Can you work these out from the model? Positions are in its coordinate system, mm. Face numbers are marked on the shaded views. A direction names the side the tool comes from. Give positions to 0.01 mm unless a question says otherwise; leave off trailing zeros. Loops run counter-clockwise (first coordinate to the right, second up) from the corner with the lowest first, then second, coordinate; pieces in that order, holes last. Notation, with made-up numbers: M -8.75,-20.5 L 49.25,-20.5 A8 cw 49.25,-9.5 Z; hole C -16.75,-0.75 d3. An arc over 180 degrees is marked long. Put each result on its own line as item: value. Start each with the question number.
1) For P1, Ø10, axis at x = 33.5, y = -88, coming from the -Z side; P2, Ø2, axis at y = -81, z = -4, coming from the +X side; P3, Ø12, axis at x = 117.5, z = 5, coming from the +Y side, each with a flat end and sliding along its axis, tell me the tip position at first contact or that it passes through.
2) Please list where these lines run through material, in increasing order: line 1 along X through (y, z) = (-70.25, 12.5); line 2 along X through (y, z) = (-75, 9); line 3 along Y through (x, z) = (90.5, 1). Write a range as from..to.
3) For the marked faces 5, 6 and 7, which set-ups out of +Z, -Z, +X, -X, +Y, -Y let a thin tool reach every point of the face, with its end or its side?
4) Imagine slicing it at C-C (x = 95). Write out the boundary of the cut face in (y, z), then the cut area to 3 significant figures.
5) Imagine slicing it at A-A (z = 12.5). Write out the boundary of the cut face in (x, y).
6) Imagine slicing it at B-B (z = -7). Write out the boundary of the cut face in (x, y).
7) If we mould it in two halves opening along Y, with no side actions, what happens to the marked faces 1, 2, 3 and 4? For each: +Y half, -Y half, draft (parallel to the pull), parting line (faces both ways), or undercut.
from build123d import *

# Parameters (mm, degrees)
SKETCH_1_W          = 170
SKETCH_1_H          = 150
EXTRUDE_1_DEPTH     = 25
CUT_EXTRUDE_1_DEPTH = 50
CHAMFER_2_SIZE      = 5
SKETCH_7_R          = 6
EXTRUDE_4_DEPTH     = 10
CHAMFER_4_SIZE      = 5
SKETCH_8_R          = 5
CUT_EXTRUDE_2_DEPTH = 229.089894559


with BuildPart() as part:
    # 草图1 → 凸台-拉伸1 (new body)
    with BuildSketch(Plane.XY):
        with Locations((85, -75)):
            Rectangle(SKETCH_1_W, SKETCH_1_H)
    extrude(amount=EXTRUDE_1_DEPTH)

    # 草图3 → 切除-拉伸1 (cut)
    with BuildSketch(Plane(origin=(0, 0, 0), x_dir=(-1, 0, 0), z_dir=(0, 0, -1))):
        with BuildLine():
            Line((-170, 0), (-105, 0))
            ThreePointArc((-105, 0), (-215.961940777, 45.961940777), (-170, -65))
            Line((-170, -65), (-170, 0))
        make_face()
        with BuildLine():
            ThreePointArc((-170, -65), (-124.038059223, -45.961940777), (-105, 0))
            Line((-105, 0), (-170, 0))
            Line((-170, 0), (-170, -65))
        make_face()
        with BuildLine():
            ThreePointArc((0, -61.846584384), (18.242646352, 52.559490104), (-85, 0))
            Line((-85, 0), (-20, 0))
            Line((-20, 0), (0, 0))
            Line((0, 0), (0, -61.846584384))
        make_face()
        with BuildLine():
            Line((-20, 0), (-85, 0))
            ThreePointArc((-85, 0), (-65.961940777, -45.961940777), (-20, -65))
            Line((-20, -65), (0, -65))
            Line((0, -65), (0, -61.846584384))
            Line((0, -61.846584384), (0, 0))
            Line((0, 0), (-20, 0))
        make_face()
        with BuildLine():
            Line((0, -150), (-85, -150))
            ThreePointArc((-85, -150), (18.242646352, -202.559490104), (0, -88.153415616))
            Line((0, -88.153415616), (0, -150))
        make_face()
        with BuildLine():
            Line((0, -88.153415616), (0, -85))
            Line((0, -85), (-20, -85))
            ThreePointArc((-20, -85), (-65.961940777, -104.038059223), (-85, -150))
            Line((-85, -150), (0, -150))
            Line((0, -150), (0, -88.153415616))
        make_face()
        with BuildLine():
            Line((-170, -150), (-170, -85))
            ThreePointArc((-170, -85), (-215.961940777, -195.961940777), (-105, -150))
            Line((-105, -150), (-170, -150))
        make_face()
        with BuildLine():
            ThreePointArc((-105, -150), (-124.038059223, -104.038059223), (-170, -85))
            Line((-170, -85), (-170, -150))
            Line((-170, -150), (-105, -150))
        make_face()
    extrude(amount=-CUT_EXTRUDE_1_DEPTH, mode=Mode.SUBTRACT)

    # 倒角2
    chamfer_2_edges = [part.edges().sort_by_distance(p)[0] for p in [
        (0, -75, 0),
        (95, 0, 0),
        (170, -75, 0),
        (95, -150, 0),
        (124.038059223, -45.961940777, 0),
        (65.961940777, -45.961940777, 0),
        (124.038059223, -104.038059223, 0),
        (65.961940777, -104.038059223, 0),
        (10, -85, 0),
        (10, -65, 0),
    ]]
    chamfer(chamfer_2_edges, length=CHAMFER_2_SIZE)

    # 草图7 → 凸台-拉伸4 (add)
    with BuildSketch(Plane(origin=(0, 0, 0), x_dir=(-1, 0, 0), z_dir=(0, 0, -1))):
        with Locations(Location((-107.5, -62.5, 0), (0, 0, 180))):
            Circle(SKETCH_7_R)
        with Locations(Location((-82.5, -62.5, 0), (0, 0, 180))):
            Circle(SKETCH_7_R)
        with Locations(Location((-82.5, -87.5, 0), (0, 0, 180))):
            Circle(SKETCH_7_R)
        with Locations(Location((-107.5, -87.5, 0), (0, 0, 180))):
            Circle(SKETCH_7_R)
    extrude(amount=EXTRUDE_4_DEPTH)

    # 倒角4
    chamfer_4_edges = [part.edges().sort_by_distance(p)[0] for p in [
        (0, -75, 25),
        (95, -150, 25),
        (170, -75, 25),
        (95, 0, 25),
        (124.038059223, -104.038059223, 25),
        (10, -85, 25),
        (65.961940777, -104.038059223, 25),
        (10, -65, 25),
        (65.961940777, -45.961940777, 25),
        (124.038059223, -45.961940777, 25),
    ]]
    chamfer(chamfer_4_edges, length=CHAMFER_4_SIZE)

    # 草图8 → 切除-拉伸2 (cut, through all)
    with BuildSketch(Plane(origin=(0, 0, 0), x_dir=(1, 0, 0), z_dir=(0, 1, 0))):
        with Locations(Location((20, -12.5, 0), (0, 0, 270))):
            Circle(SKETCH_8_R)
    extrude(amount=-CUT_EXTRUDE_2_DEPTH, mode=Mode.SUBTRACT)


solid = part.part
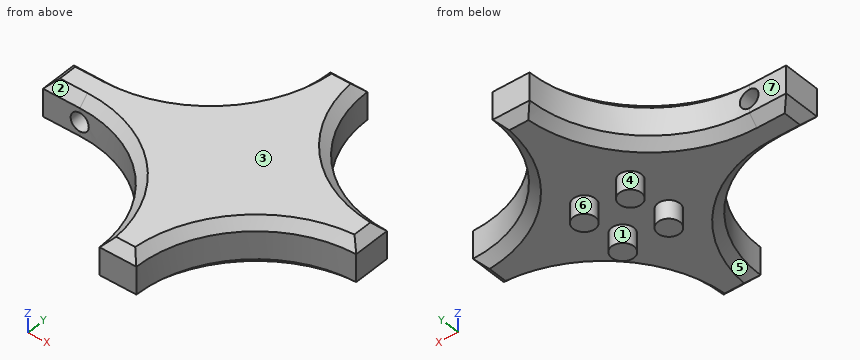
Recorded:
1. P1: z = 1.55
1. P2: x = 109.9
1. P3: y = -28.33
2. line 1: 0..15, 25..170
2. line 2: 0..16.43, 23.57..170
2. line 3: -146..-4
3. face 5: -Z, -X, -Y
3. face 6: -Z
3. face 7: +Z, -Z, -X, +Y
4. outline: M -150,5 L -145,0 L -5,0 L 0,5 L 0,20 L -5,25 L -145,25 L -150,20 Z
4. area: 3,700 mm²
5. outline: M 0,-85 L 15,-85 L 15,-65 L 0,-65 Z; M 25,-85.19 A65 cw 85,-150 L 105,-150 A65 cw 170,-85 L 170,-65 A65 cw 105,0 L 85,0 A65 cw 25,-64.81 Z
6. outline: C 82.5,-87.5 d12; C 82.5,-62.5 d12; C 107.5,-87.5 d12; C 107.5,-62.5 d12
7. face 1: undercut
7. face 2: -Y half
7. face 3: draft
7. face 4: undercut
